from build123d import *

# Parameters (mm, degrees)
SKETCH_W             = 124
SKETCH_H             = 124
PAD_DEPTH            = 2
POCKET_DEPTH         = 2.001
POCKET_DEPTH_BACK    = -2.001
POCKET001_DEPTH      = 2.001
POCKET001_DEPTH_BACK = -2.001
SKETCH006_W          = 150
SKETCH006_H          = 77
POCKET002_DEPTH      = 2.001
POCKET002_DEPTH_BACK = -2.001
POCKET003_DEPTH      = 2.001
POCKET003_DEPTH_BACK = -2.001
FILLET_R             = 2
FILLET001_R          = 2
FILLET002_R          = 0.5
SKETCH008_W          = 5
SKETCH008_H          = 10
PAD001_DEPTH         = 3
CHAMFER_SIZE         = 2.99


with BuildPart() as part:
    # Sketch → Pad (new body, symmetric)
    with BuildSketch(Plane.XY):
        with Locations((0, 62)):
            Rectangle(SKETCH_W, SKETCH_H)
    extrude(amount=PAD_DEPTH, both=True)

    # Sketch004 → Pocket (cut, two sides)
    with BuildSketch(Plane.XY) as pocket_sk:
        Polygon((-58, 5), (-62, 5), (-62, 15), (-58, 15), (-58, 80), (-62, 80), (-62, 90), (-58, 90), (-58, 124), (-88, 124), (-88, 0), (-58, 0), align=None)
        Polygon((58, 5), (62, 5), (62, 15), (58, 15), (58, 80), (62, 80), (62, 90), (58, 90), (58, 124), (88, 124), (88, 0), (58, 0), align=None)
    extrude(amount=-POCKET_DEPTH, mode=Mode.SUBTRACT)
    extrude(pocket_sk.sketch, amount=-POCKET_DEPTH_BACK, mode=Mode.SUBTRACT)

    # Sketch005 → Pocket001 (cut, two sides)
    with BuildSketch(Plane.XY) as pocket001_sk:
        Polygon((-60, 120), (-40, 120), (-40, 124), (-30, 124), (-30, 120), (30, 120), (30, 124), (40, 124), (40, 120), (60, 120), (60, 130), (-60, 130), align=None)
    extrude(amount=-POCKET001_DEPTH, mode=Mode.SUBTRACT)
    extrude(pocket001_sk.sketch, amount=-POCKET001_DEPTH_BACK, mode=Mode.SUBTRACT)

    # Sketch006 → Pocket002 (cut, two sides)
    with BuildSketch(Plane.XY) as pocket002_sk:
        with Locations((0, 38.5)):
            Rectangle(SKETCH006_W, SKETCH006_H)
    extrude(amount=-POCKET002_DEPTH, mode=Mode.SUBTRACT)
    extrude(pocket002_sk.sketch, amount=-POCKET002_DEPTH_BACK, mode=Mode.SUBTRACT)

    # Sketch007 → Pocket003 (cut, two sides)
    with BuildSketch(Plane.XY) as pocket003_sk:
        with BuildLine():
            ThreePointArc((4, 90.26136), (-49, 71), (4, 51.73864))
            Line((4, 90.26136), (4, 51.73864))
        make_face()
    extrude(amount=-POCKET003_DEPTH, mode=Mode.SUBTRACT)
    extrude(pocket003_sk.sketch, amount=-POCKET003_DEPTH_BACK, mode=Mode.SUBTRACT)

    # Fillet
    fillet_edges = [part.edges().sort_by_distance(p)[0] for p in [
        (-48.393877, 77, 0),
        (4, 90.26136, 0),
        (4, 77, 0),
        (58, 77, 0),
        (-58, 77, 0),
    ]]
    fillet(fillet_edges, radius=FILLET_R)

    # Fillet001
    fillet001_edges = [part.edges().sort_by_distance(p)[0] for p in [
        (58, 120, 0),
        (-58, 120, 0),
    ]]
    fillet(fillet001_edges, radius=FILLET001_R)

    # Fillet002
    fillet002_edges = [part.edges().sort_by_distance(p)[0] for p in [
        (-58, 80, 0),
        (-62, 80, 0),
        (-62, 90, 0),
        (-58, 90, 0),
        (-40, 120, 0),
        (-40, 124, 0),
        (-30, 124, 0),
        (-30, 120, 0),
        (30, 120, 0),
        (30, 124, 0),
        (40, 124, 0),
        (40, 120, 0),
        (58, 90, 0),
        (62, 90, 0),
        (62, 80, 0),
        (58, 80, 0),
    ]]
    fillet(fillet002_edges, radius=FILLET002_R)

    # Sketch008 (on DatumPlane) → Pad001 (join)
    with BuildSketch(Plane.XY.offset(-2)):
        with Locations((-52.5, 77)):
            Rectangle(SKETCH008_W, SKETCH008_H)
        with Locations((8.5, 77)):
            Rectangle(SKETCH008_W, SKETCH008_H)
        with Locations((53.5, 77)):
            Rectangle(SKETCH008_W, SKETCH008_H)
    extrude(amount=-PAD001_DEPTH)

    # Chamfer
    chamfer_edges = [part.edges().sort_by_distance(p)[0] for p in [
        (-52.5, 82, -2),
        (8.5, 82, -2),
        (53.5, 82, -2),
    ]]
    chamfer(chamfer_edges, length=CHAMFER_SIZE)


solid = part.part
Design review of the part built by this model. Coordinates are the model's own, in mm. A direction names the side the tool comes from. Coordinates: 2 decimals unless noted, no trailing zeros. Write each loop counter-clockwise with the first axis right and the second up, starting at its lowest first coordinate (ties: lowest second). Pieces come first, ordered by that corner, then holes. Notation, with made-up numbers: (-8, 43.25) - (6, 43.25) arc R14 cw to (6, 70.25) - close; hole circle Ø3 at (48, 87.25). An arc over 180 degrees is marked (long way). One line per item, written item: value.
1) To check wall thickness, follow probe 1 along X at (y, z) = (78, -3.75); probe 2 along Z at (x, y) = (39, 90); probe 3 along Y at (x, z) = (19, -0.25). State the ranges of each line that lie inside material, in increasing order.
Answer sheet:
probe 1: x = -55 to -50, 6 to 11, 51 to 56
probe 2: z = -2 to 2
probe 3: y = 77 to 120
2) Add section A-A (z = -3.5). State the section outline as (x, y) points, plus the area to 3 significant figures.
Answer sheet:
outline: (-55, 72) - (-50, 72) - (-50, 83.49) - (-55, 83.49) - close; (6, 72) - (11, 72) - (11, 83.49) - (6, 83.49) - close; (51, 72) - (56, 72) - (56, 83.49) - (51, 83.49) - close
area: 172 mm2
3) Add section D-D (y = 87). State the section outline as (x, z) points.
Answer sheet:
outline: (-62, -2) - (-44.38, -2) - (-44.38, 2) - (-62, 2) - close; (4, -2) - (62, -2) - (62, 2) - (4, 2) - close
4) Add section C-C (x = 38). State the section outline as (y, z) points, plus the area to 3 significant figures.
Answer sheet:
outline: (77, -2) - (124, -2) - (124, 2) - (77, 2) - close
area: 188 mm2
5) Mouldability with a two-part tool opening along X and no side actions: class faces 1 (the face through (11, 78, -3)), 2 (the face through (8, 72, -3)), 3 (the face through (-62, 85, 0)) as +X half, -X half, draft (parallel to the pull), parting line (faces both ways), or undercut.
Answer sheet:
face 1: undercut
face 2: draft
face 3: -X half
6) For faces 4 (the face through (-55, 78, -3)), 5 (the face through (-60, 80, 0)), 6 (the face through (58, 104, 0)), 7 (the face through (-40, 122, 0)), 8 (the face through (-53, 75, -2)), list the 3-axis set-ups (+Z, -Z, +X, -X, +Y, -Y) from which the entire face can be reached by the end or side of a thin tool; tool diameter is ignored.
Answer sheet:
face 4: -Z, -X, +Y, -Y
face 5: +Z, -Z, -X, -Y
face 6: +Z, -Z, +X, +Y
face 7: +Z, -Z, -X, +Y
face 8: +Z, +X, -X, -Y
7) Insertion check: pin 1 (0.9 mm diameter, centred on y = 79.5, z = -4, fed in from -X); pin 2 (1.2 mm diameter, centred on x = 47, z = 0.5, fed in from +Y); pin 3 (2.5 mm diameter, centred on y = 122.5, z = 0.5, fed in from +X). Each pin has a flat end and moves straight along its axis. Give the tip position at first contact, or say it passes through.
Answer sheet:
pin 1: stops at x = -55
pin 2: stops at y = 120
pin 3: stops at x = 40
8) Add section B-B (y = 99). State the section outline as (x, z) points.
Answer sheet:
outline: (-58, -2) - (-29.77, -2) - (-29.77, 2) - (-58, 2) - close; (-8.23, -2) - (58, -2) - (58, 2) - (-8.23, 2) - close
